Autodesk Inventor part; units mm, degrees
ref_plane "YZ Plane" through (0, 0, 0) normal (1, 0, 0) x (0, 1, 0)
ref_plane "XZ Plane" through (0, 0, 0) normal (0, 1, 0) x (-1, 0, 0)
ref_plane "XY Plane" through (0, 0, 0) normal (0, 0, 1) x (1, 0, 0)
sketch "Sketch1" plane through (0, 0, 0) normal (0, 1, 0) x (-1, 0, 0)
  line L0 (0, 0) -> (0, -253.429) construction
  line L1 (5, 0) -> (5, -253.429)
  line L2 (-5, -253.429) -> (-5, 0)
  arc A0 (5, 0) -> (-5, 0) centre (0, 0) ccw
  arc A1 (-5, -253.429) -> (5, -253.429) centre (0, -253.429) ccw
  circle A2 centre (0, 0) radius 1.65
  circle A3 centre (0, -253.429) radius 1.65
  arc A4 (5, -253.429) -> (5, 0) centre (-1489.6382, -126.7145) ccw
  arc A5 (-5, -253.429) -> (-5, 0) centre (-1499.6382, -126.7145) ccw
  circle A6 centre (5.3131, -141.429) radius 1.65
  point P0 (0, -126.7145)
  dimension "d0" = 3.3
  dimension "d1" = 3.3
  dimension "d2" = 10
  dimension "d3" = 253.429
  dimension "d16" = 1500
  dimension "d17" = 1500
  dimension "d18" = 3.3
  dimension "d19" = 112
extrude "Extrusion1" add sketch "Sketch1" along normal blind 6 contours A4 L1 A6 | L1 A6 A1 A5 A0
sketch "Sketch2" plane through (0, 6, 0) normal (0, 1, 0) x (1, 0, 0)
  line L0 (-23.0122, 130.7764) -> (18.8584, 130.7764)
  line L1 (18.8584, 130.7764) -> (18.8584, -10.1345)
  line L2 (18.8584, -10.1345) -> (-23.0122, -10.1345)
  line L3 (-23.0122, -10.1345) -> (-23.0122, 130.7764)
  line L4 (-71.0561, 282.155) -> (73.8808, 282.155)
  line L5 (73.8808, 282.155) -> (73.8808, -35.6326)
  line L6 (73.8808, -35.6326) -> (-71.0561, -35.6326)
  line L7 (-71.0561, -35.6326) -> (-71.0561, 282.155)
  point P0 (0, 0)
extrude "Extrusion2" cut sketch "Sketch2" against normal blind 10
properties part number "Part_5_p1"
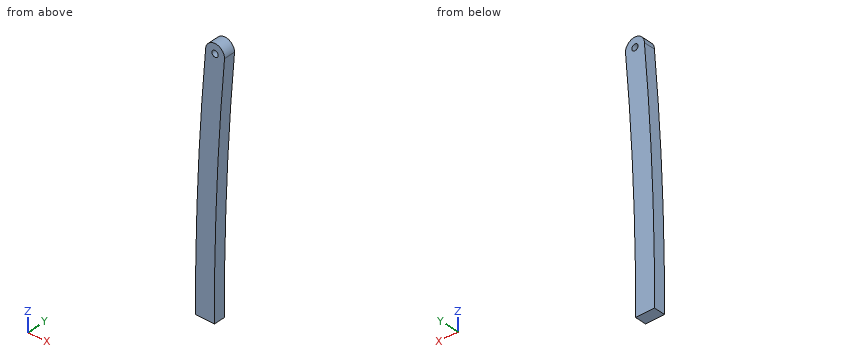
Geometry: final body of the model. Coordinates: model frame, mm. Round coordinates to 2 decimals unless told otherwise and drop trailing zeros. Write each loop counter-clockwise with the first axis right and the second up, starting at its lowest first coordinate (ties: lowest second). Pieces come first, ordered by that corner, then holes. Notation, with made-up numbers: (42.25, -31) -> (76.25, -31) arc R18 ccw to (76.25, -9) -> close; hole circle Ø9 at (-22.75, -20.5). An arc over 180 degrees is marked (long way). Use CSV: the item, a comma, the result in double quotes. Start each with the question number.
Q1. Line query: L1, parallel to Z at x = -4, y = 3; L2, parallel to X at y = 3.8, z = -37; L3, parallel to X at y = 0.45, z = -79. Output: solid intervals per line, ascending.
Q2. First-contact query: pin 1 Ø4.5 at (x, z) = (0, 0) entering from +Y; pin 2 Ø1 at (y, z) = (1.5, -14) entering from -X; pin 3 Ø3 at (x, y) = (-5.5, 2) entering from +Z; pin 4 Ø1 at (x, y) = (1, 5) entering from +Z. Flat tips, straight axial feed; report the tip coordinate or a pass-through.
Q3. Section B-B (z = -91.5). Return loops of the section in (x, y), plus the area to 3 significant figures.
Q4. Section A-A (y = 4.9). Return loops of the section in (x, z), plus the area to 3 significant figures.
Result sheet:
1,L1,"-130.78 to 3"
1,L2,"-7.68 to 2.32"
1,L3,"-9.6 to 0.4"
2,pin 1,"y = 6"
2,pin 2,"x = -6.16"
2,pin 3,"z = 3"
2,pin 4,"z = 4.97"
3,outline,"(-9.95, 0) -> (0.05, 0) -> (0.05, 6) -> (-9.95, 6) -> close"
3,area,"60.0 mm²"
4,outline,"(-10.36, -130.78) -> (-0.36, -130.78) arc R1500 cw to (5, 0) arc R5 ccw to (-5, 0) arc R1500 ccw to start; hole circle Ø3.3 at (0, 0)"
4,area,"1,340 mm²"
